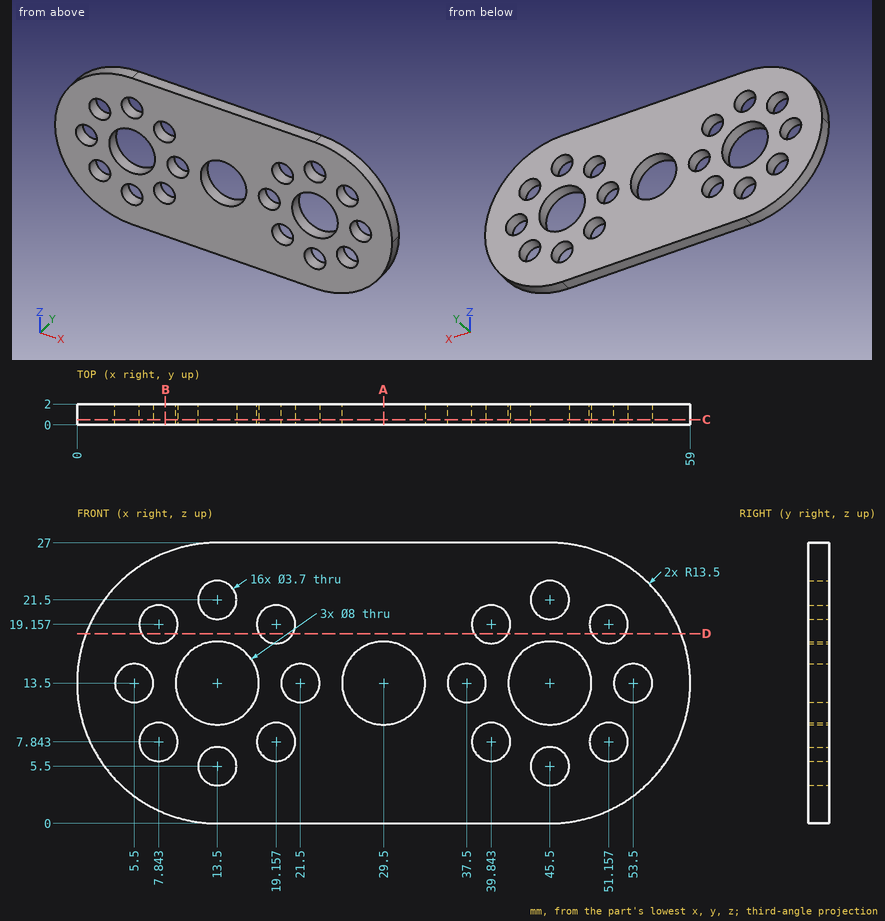
Print and shaded views of the part. All mm, measured from the part's lowest x, y and z. Give positions to 0.01 mm unless a question says otherwise; leave off trailing zeros. Loops run counter-clockwise (first coordinate to the right, second up) from the corner with the lowest first, then second, coordinate; pieces in that order, holes last. Notation, with made-up numbers: M 43.5,-22.75 L 62.5,-22.75 A12 cw 62.5,-0.75 Z; hole C 76,42 d1. An arc over 180 degrees is marked long. Write each question's results on one line, items separated by ' | '.
Q1. Band-saw the part on D-D on z = 18.25. Write the cut outline in (x, y).
Geometry check:
outline: M 0.86,0 L 6.23,0 L 6.23,2 L 0.86,2 Z; M 9.46,0 L 17.54,0 L 17.54,2 L 9.46,2 Z; M 20.77,0 L 38.23,0 L 38.23,2 L 20.77,2 Z; M 41.46,0 L 49.54,0 L 49.54,2 L 41.46,2 Z; M 52.77,0 L 58.14,0 L 58.14,2 L 52.77,2 Z
Q2. Band-saw the part on B-B on x = 8.5. Write the cut outline in (y, z), and give its area (3 significant figures).
Geometry check:
outline: M 0,0.96 L 2,0.96 L 2,6.11 L 0,6.11 Z; M 0,9.57 L 2,9.57 L 2,17.43 L 0,17.43 Z; M 0,20.89 L 2,20.89 L 2,26.04 L 0,26.04 Z | area: 36.3 mm²
Q3. Probe probe 1 along Z at (x, y) = (46, 0.3); probe 2 along Z at (x, y) = (19.5, 0.5) (1 decimal); probe 3 along Z at (x, y) = (52.5, 1.7) (1 decimal). List the from-to ranges inside material, lowest first.
Geometry check:
probe 1: z = 0.01 to 3.72, 7.28 to 9.53, 17.47 to 19.72, 23.28 to 26.99 | probe 2: z = 0 to 6, 9.7 to 17.3, 21 to 27 | probe 3: z = 2 to 6.6, 9.1 to 11.9, 15.1 to 17.9, 20.4 to 25
Q4. Band-saw the part on A-A on x = 29.5. Write the cut outline in (y, z).
Geometry check:
outline: M 0,0 L 2,0 L 2,9.5 L 0,9.5 Z; M 0,17.5 L 2,17.5 L 2,27 L 0,27 Z
Q5. Flat gauge pin, fed straight in: P1, Ø2, axis at x = 40, z = 19, coming from the +Y side. Where does the tip first touch, or does it go through?
Geometry check:
P1: passes through
Q6. Band-saw the part on C-C on y = 0.5. Give the number of separate pieces and of enclosed holes in the cut face, and give its area (3 significant figures).
Geometry check:
separate pieces: 1 | enclosed holes: 19 | area: 1,110 mm²
